Study the drawing (mm; zero at the part's minimum x, y, z) and answer. A direction names the side the tool comes from. Coordinates: 2 decimals unless noted, no trailing zeros. Loops run counter-clockwise (first coordinate to the right, second up) from the corner with the lowest first, then second, coordinate; pieces in that order, holes last.
Q1. Section A-A (z = 43) is taken. Give the vertices of the cut face in (x, y).
Q2. Section C-C (y = 59) is taken. Give the vertices of the cut face in (x, z).
Q3. Flat-ended cylindrical pins translate along their axes: P1, Ø4, axis at y = 49.5, z = 46, coming from the +X side; P2, Ø21, axis at x = 107.5, z = 36, coming from the +Y side; P3, Ø5, axis at x = 107.5, y = 14.5, coming from the +Z side. Find the tip coordinate at first contact, or state that the pin passes through.
Q4. Section B-B (x = 93) is taken. Give the vertices of the cut face in (y, z), then the cut area to 3 significant figures.
Q5. Straight lines are drawn through the part: line 1 (X direction, y = 3, z = 4.5); line 2 (Y direction, x = 72, z = 24); line 3 (Y direction, x = 107, z = 26.5). For each, find the intervals that lie inside material, in ascending order.
Q6. The mould has two halves that part along X. Classify the marked faces 1, 2 and 3: pulls with the +X half, pulls with the -X half, needs draft (parallel to the pull), parting line crosses it, or undercut.
Q7. Which of the six approach directions +Z, -Z, +X, -X, +Y, -Y give full straight-line access (tool end or side, diameter ignored) to the marked faces 4, 5 and 6?
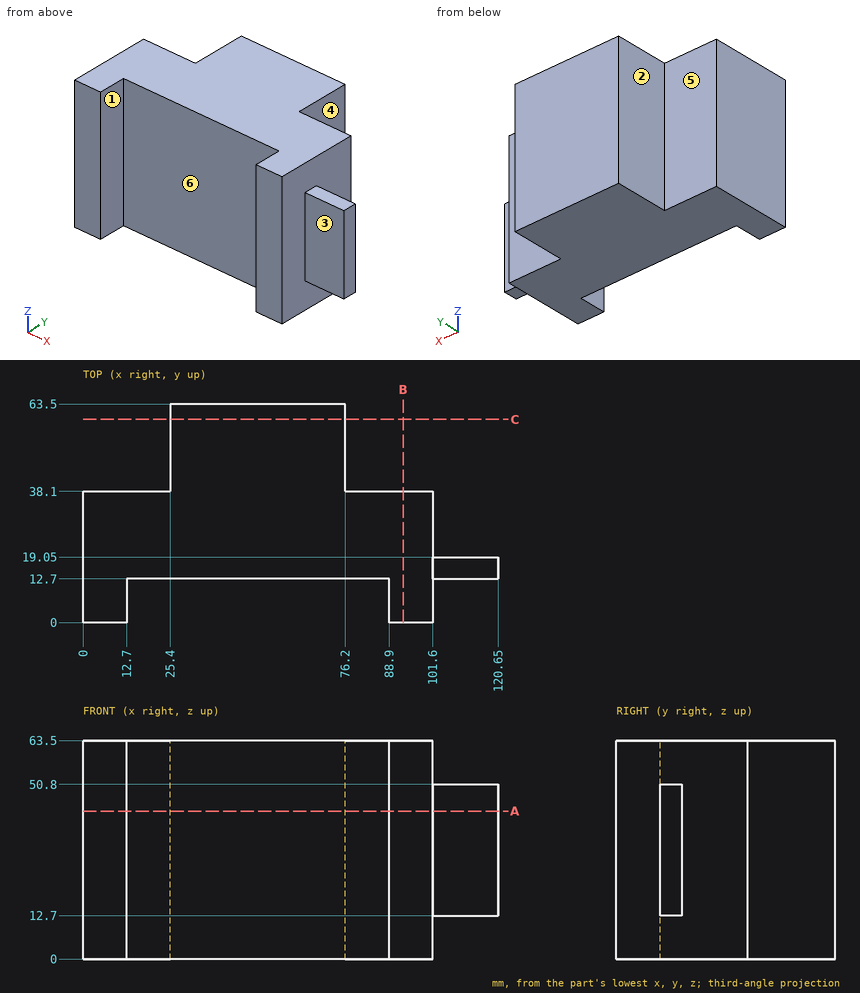
Numbers:
1. outline: (0, 0) - (12.7, 0) - (12.7, 12.7) - (88.9, 12.7) - (88.9, 0) - (101.6, 0) - (101.6, 12.7) - (120.65, 12.7) - (120.65, 19.05) - (101.6, 19.05) - (101.6, 38.1) - (76.2, 38.1) - (76.2, 63.5) - (25.4, 63.5) - (25.4, 38.1) - (0, 38.1) - close
2. outline: (25.4, 0) - (76.2, 0) - (76.2, 63.5) - (25.4, 63.5) - close
3. P1: stops at x = 76.2
3. P2: stops at y = 38.1
3. P3: stops at z = 50.8
4. outline: (0, 0) - (38.1, 0) - (38.1, 63.5) - (0, 63.5) - close
4. area: 2,420 mm2
5. line 1: x = 0 to 12.7, 88.9 to 101.6
5. line 2: y = 12.7 to 63.5
5. line 3: y = 12.7 to 19.05
6. face 1: undercut
6. face 2: pulls with the -X half
6. face 3: needs draft
7. face 4: +Z, -Z, +X, +Y
7. face 5: +Z, -Z, -X, +Y
7. face 6: +Z, -Z, -Y
